```python
from build123d import *

# Parameters (mm, degrees)
SKETCH_1_W                  = 30
SKETCH_1_H                  = 15
EXTRUDE_1_DEPTH             = 3
EXTRUDE_2_DEPTH             = 3
FILLET_1_R                  = 4
FILLET_2_R                  = 3
FILLET_5_R                  = 4
FILLET_6_R                  = 4
SKETCH_3_R                  = 1.05
CUT_EXTRUDE_1_DEPTH         = 3
SKETCH_4_R                  = 1.505
CUT_EXTRUDE_2_DEPTH         = 40
EXTRUDE_START               = -11
EXTRUDE_3_OUTLINE_W         = 5.656854249
EXTRUDE_3_OUTLINE_H         = 3
EXTRUDE_3_DEPTH             = 2.161165235
SKETCH_7_R                  = 1.5
CUT_EXTRUDE_3_DEPTH         = 40
FILLET_7_R                  = 10
FILLET_8_R                  = 10
SKETCH_8_R                  = 1.5
CUT_EXTRUDE_4_DEPTH         = 40
EXTRUDE_4_DEPTH             = 3
HOLE_WIZARD_M3_1_AT_2_COUNT = 2
HOLE_WIZARD_M3_1_AT_2_PITCH = 26.570660511
HOLE_WIZARD_M3_1_AT_3_COUNT = 2
HOLE_WIZARD_M3_1_AT_3_PITCH = 31.5
FILLET_9_R                  = 4
SKETCH_12_R                 = 1.5
CUT_EXTRUDE_5_DEPTH         = 20.5


with BuildPart() as part:
    # 草图1 → 凸台-拉伸1 (new body)
    with BuildSketch(Plane.XY):
        Rectangle(SKETCH_1_W, SKETCH_1_H)
    extrude(amount=EXTRUDE_1_DEPTH)

    # 草图2 → 凸台-拉伸2 (add)
    with BuildSketch(Plane.XY.offset(3)):
        Polygon((-15, 7.5), (-15, 16), (-24, 16), (-24, 24), (-33, 24), (-33, -15.5), (-24, -15.5), (-24, -7.5), (-15, -7.5), align=None)
    extrude(amount=-EXTRUDE_2_DEPTH)

    # 圆角1
    fillet_1_edges = [part.edges().sort_by_distance(p)[0] for p in [
        (-24, 24, 1.5),
        (-33, 24, 1.5),
    ]]
    fillet(fillet_1_edges, radius=FILLET_1_R)

    # 圆角2
    fillet_2_edges = [part.edges().sort_by_distance(p)[0] for p in [
        (-24, 16, 1.5),
    ]]
    fillet(fillet_2_edges, radius=FILLET_2_R)

    # 圆角5
    fillet_5_edges = [part.edges().sort_by_distance(p)[0] for p in [
        (-33, -15.5, 1.5),
        (-24, -15.5, 1.5),
    ]]
    fillet(fillet_5_edges, radius=FILLET_5_R)

    # 圆角6
    fillet_6_edges = [part.edges().sort_by_distance(p)[0] for p in [
        (-24, -7.5, 1.5),
    ]]
    fillet(fillet_6_edges, radius=FILLET_6_R - 0.0001)  # a hair under: the kernel refuses the full size

    # 草图3 → 切除-拉伸1 (cut)
    with BuildSketch(Plane.XY.offset(3)):
        with Locations((-13.95, 7.5)):
            Circle(SKETCH_3_R)
    extrude(amount=-CUT_EXTRUDE_1_DEPTH, mode=Mode.SUBTRACT)

    # 草图4 → 切除-拉伸2 (cut)
    with BuildSketch(Plane.XY.offset(3)):
        with Locations((-29, 20)):
            Circle(SKETCH_4_R)
    extrude(amount=-CUT_EXTRUDE_2_DEPTH, mode=Mode.SUBTRACT)

    # 凸台-拉伸3: read off the stored shape, not the designer's step
    # 凸台-拉伸3 outline → 凸台-拉伸3 (add)
    with BuildSketch(Plane(origin=(0, 0, 0), x_dir=(0.7071067811865471, 0.707106781186548, 0), z_dir=(0.707106781186548, -0.707106781186547, 0)).offset(EXTRUDE_START)):
        with Locations((-22.273863608, 1.5)):
            Rectangle(EXTRUDE_3_OUTLINE_W, EXTRUDE_3_OUTLINE_H)
    extrude(amount=EXTRUDE_3_DEPTH)

    # 草图7 → 切除-拉伸3 (cut)
    with BuildSketch(Plane.XY.offset(3)):
        with Locations((-20, -5)):
            Circle(SKETCH_7_R)
    extrude(amount=-CUT_EXTRUDE_3_DEPTH, mode=Mode.SUBTRACT)

    # 圆角7
    fillet_7_edges = [part.edges().sort_by_distance(p)[0] for p in [
        (-20, -7.5, 1.5),
    ]]
    fillet(fillet_7_edges, radius=FILLET_7_R)

    # 圆角8
    # the kernel refuses this fillet: 10 mm, written as the material it adds along each edge
    with BuildSketch(Plane(origin=(-24, -11.5, 3), x_dir=(0.7071067811080579, 0.7071067812650372, 0), z_dir=(0, 0, -1))) as fillet_8_piece_1:
        with BuildLine():
            CenterArc((3.037620293, 9.883358261), FILLET_8_R, 245.228316877, 16.01201465)
            Line((-1.152413577, 0.803511557), (-1.236214254, 0.621914623))
            ThreePointArc((-1.236214254, 0.621914623), (-0.655043014, 0.288687166), (-0.141421356, -0.141421356))
            Line((-0.141421356, -0.141421356), (0, -0.2))
            ThreePointArc((0, -0.2), (0.757359313, -0.2), (1.484260592, -0.197667165))
            Line((1.484260592, -0.197667165), (1.514718626, 0))
        make_face()
    extrude(amount=3)

    # 草图8 → 切除-拉伸4 (cut)
    with BuildSketch(Plane.XY.offset(3)):
        with Locations((-29, -11.5)):
            Circle(SKETCH_8_R)
    extrude(amount=-CUT_EXTRUDE_4_DEPTH, mode=Mode.SUBTRACT)

    # 草图11 → 凸台-拉伸4 (add)
    with BuildSketch(Plane.XY.offset(3)):
        with BuildLine():
            Line((-15.857864376, -7.5), (-22.928932188, -10.428932188))
            ThreePointArc((-22.928932188, -10.428932188), (-19.6846987, -8.261204675), (-15.857864376, -7.5))
        make_face()
    extrude(amount=-EXTRUDE_4_DEPTH)

    # 草图10 → M3 十字槽半沉头木螺钉的锥形沉头孔1 (revolve, cut)
    with BuildSketch(Plane(origin=(-29, 20, 3), x_dir=(0, -1, 0), z_dir=(1, 0, 0))):
        Polygon((0, 0), (0, 3), (1.5, 3), (1.5, 1.8), (3.3, 0), align=None)
    hole_wizard_m3_1 = revolve(axis=Axis((-29, 20, 9.35), (0, 0, -1)), mode=Mode.SUBTRACT)

    # M3 十字槽半沉头木螺钉的锥形沉头孔1 at 2: M3 十字槽半沉头木螺钉的锥形沉头孔1 ×2
    with Locations(*[Vector(0.33871946827274174, -0.9408874118687268, 0) * (i * HOLE_WIZARD_M3_1_AT_2_PITCH) for i in range(1, HOLE_WIZARD_M3_1_AT_2_COUNT)]):
        add(hole_wizard_m3_1, mode=Mode.SUBTRACT)

    # M3 十字槽半沉头木螺钉的锥形沉头孔1 at 3: M3 十字槽半沉头木螺钉的锥形沉头孔1 ×2
    with Locations(*[(0, -i * HOLE_WIZARD_M3_1_AT_3_PITCH, 0) for i in range(1, HOLE_WIZARD_M3_1_AT_3_COUNT)]):
        add(hole_wizard_m3_1, mode=Mode.SUBTRACT)

    # 圆角9
    fillet_9_edges = [part.edges().sort_by_distance(p)[0] for p in [
        (-15.857864377, -7.5, 1.5),
        (-22.928932188, -10.428932188, 1.5),
    ]]
    fillet(fillet_9_edges, radius=FILLET_9_R)

    # 草图12 → 切除-拉伸5 (cut, symmetric)
    with BuildSketch(Plane.XY.offset(3)):
        with Locations(Location((0, -2.5, 0), (0, 0, 180))):
            Circle(SKETCH_12_R)
    extrude(amount=CUT_EXTRUDE_5_DEPTH, both=True, mode=Mode.SUBTRACT)


solid = part.part
```
Input: part model. Units: mm. Frame: model coordinates. A direction names the side the tool comes from. Round coordinates to 2 decimals unless told otherwise and drop trailing zeros. Order: outer loops, then holes, each group sorted by start corner. A loop starts at its lowest first (then second) coordinate and runs counter-clockwise, first axis right, second up. Notation, with made-up numbers: (-6.5, 67) - (49.5, 67) arc R11 ccw to (49.5, 82) - close; hole circle Ø5 at (27, 38). An arc over 180 degrees is marked (long way). Answer in a Markdown table with one row per item.
Item 1: Pin query (flat end, axial travel): pin 1 (5 mm diameter, centred on x = -20, y = -5, fed in from +Z); pin 2 (1.5 mm diameter, centred on x = 1, z = 2, fed in from -Y); pin 3 (1.5 mm diameter, centred on y = 12.5, z = 2, fed in from +X). Return the tip coordinate at first contact, or that it passes through.
Model answer:
| item | result |
|---|---|
| pin 1 | stops at z = 2.2 |
| pin 2 | stops at y = -7.5 |
| pin 3 | stops at x = -15 |
Item 2: Mould query, pull axis Y, two halves, no side actions, for faces 4 (the cylindrical face through (-13.97, 6.45, 1.52)), 5 (the cylindrical face through (-31.859, -14.297, 1.479)), 6 (the flat face through (15, 0, 1)), 7 (the cylindrical face through (0, -1, 2)). Classes: released by +Y, released by -Y, zero draft, split by the parting line, or undercut.
Model answer:
| item | result |
|---|---|
| face 4 | released by +Y |
| face 5 | released by -Y |
| face 6 | zero draft |
| face 7 | undercut |
Item 3: Line query: line 1 (Y direction, x = -29, z = 0.95) (3 decimals); line 2 (X direction, y = -5, z = 0.6); line 3 (Y direction, x = 0, z = 1.4). Output: solid intervals per line, ascending.
Model answer:
| item | result |
|---|---|
| line 1 | y = -15.5 to -13, -10 to 18.495, 21.505 to 24 |
| line 2 | x = -33 to -21.5, -18.5 to 15 |
| line 3 | y = -7.5 to -4, -1 to 7.5 |
Item 4: Section query A-A (z = 2.35). Return the cut outline in (x, y), then the cut area to 3 significant figures.
Model answer:
| item | result |
|---|---|
| outline | (-33, -11.5) arc R4 ccw to (-29, -15.5) - (-28, -15.5) arc R4 ccw to (-24.25, -12.88) arc R10 cw to (-23.79, -11.83) arc R4 cw to (-21.75, -9.94) - (-16.59, -7.8) arc R4 cw to (-15.06, -7.5) - (15, -7.5) - (15, 7.5) - (-12.9, 7.5) arc R1.05 cw to (-15, 7.5) - (-15, 16) - (-21, 16) arc R3 cw to (-24, 19) - (-24, 20) arc R4 ccw to (-28, 24) - (-29, 24) arc R4 ccw to (-33, 20) - close; hole circle Ø5.3 at (-29, -11.5); hole circle Ø5.3 at (-29, 20); hole circle Ø5.3 at (-20, -5); hole circle Ø3 at (0, -2.5) |
| area | 945 mm² |
Item 5: Section query C-C (x = -20). Return the cut outline in (y, z).
Model answer:
| item | result |
|---|---|
| outline | (-9.22, 0) - (-6.5, 0) - (-6.5, 1.2) - (-8.3, 3) - (-9.22, 3) - close; (-3.5, 0) - (16, 0) - (16, 3) - (-1.7, 3) - (-3.5, 1.2) - close |
Item 6: Section query B-B (x = 0). Return the cut outline in (y, z).
Model answer:
| item | result |
|---|---|
| outline | (-7.5, 0) - (-4, 0) - (-4, 3) - (-7.5, 3) - close; (-1, 0) - (7.5, 0) - (7.5, 3) - (-1, 3) - close |
Item 7: Section query D-D (y = 8.5). Return the cut outline in (x, z), then the cut area to 3 significant figures.
Model answer:
| item | result |
|---|---|
| outline | (-33, 0) - (-15, 0) - (-15, 3) - (-33, 3) - close |
| area | 54.0 mm² |
Item 8: Reachability of faces 1 (the flat face through (0, -7.5, 2)), 2 (the cylindrical face through (-31.859, 22.797, 1.479)), 3 (the flat face through (-15, 12, 2)) from +Z, -Z, +X, -X, +Y, -Y: full face, straight path, thin tool, end or side. Return the list, or none.
Model answer:
| item | result |
|---|---|
| face 1 | +Z, -Z, +X, -Y |
| face 2 | +Z, -Z, -X, +Y |
| face 3 | +Z, -Z, +X, +Y |
